from build123d import *

# Parameters (mm, degrees)
SKETCH_W        = 165
SKETCH_H        = 45
PAD_DEPTH       = 22
SKETCH001_W     = 133
SKETCH001_H     = 41
POCKET_DEPTH    = 20
SKETCH002_W     = 26
SKETCH002_H     = 41
POCKET001_DEPTH = 20
SKETCH003_W     = 42
SKETCH003_H     = 47
PAD001_DEPTH    = 2
SKETCH008_W     = 42
SKETCH008_H     = 25
PAD002_DEPTH    = 6
SKETCH005_W     = 30
SKETCH005_H     = 13
POCKET002_DEPTH = 8.001
SKETCH009_R     = 1.5
POCKET003_DEPTH = 8.001
SKETCH007_R     = 2.5
POCKET004_DEPTH = 5


with BuildPart() as part:
    # Sketch → Pad (new body)
    with BuildSketch(Plane.XY):
        with Locations((82.5, 22.5)):
            Rectangle(SKETCH_W, SKETCH_H)
    extrude(amount=PAD_DEPTH)

    # Sketch001 → Pocket (cut)
    with BuildSketch(Plane.XY.offset(22)):
        with Locations((68.54825, 22.488898)):
            Rectangle(SKETCH001_W, SKETCH001_H)
    extrude(amount=-POCKET_DEPTH, mode=Mode.SUBTRACT)

    # Sketch002 → Pocket001 (cut)
    with BuildSketch(Plane.XY.offset(22)):
        with Locations((149.979632, 22.458033)):
            Rectangle(SKETCH002_W, SKETCH002_H)
    extrude(amount=-POCKET001_DEPTH, mode=Mode.SUBTRACT)

    # Sketch003 → Pad001 (new body)
    with BuildSketch(Plane(origin=(0, 45, 0), x_dir=(-1, 0, 0), z_dir=(0, 1, 0))):
        with Locations((-55.599999, 23.509954)):
            Rectangle(SKETCH003_W, SKETCH003_H)
    extrude(amount=PAD001_DEPTH)

    # Sketch008 → Pad002 (new body)
    with BuildSketch(Plane.XZ.offset(-45)):
        with Locations((55.598549, 34.508675)):
            Rectangle(SKETCH008_W, SKETCH008_H)
    extrude(amount=PAD002_DEPTH)

    # Sketch005 → Pocket002 (cut, through all)
    with BuildSketch(Plane.XZ.offset(-39)):
        with Locations((55.035654, 34.372233)):
            Rectangle(SKETCH005_W, SKETCH005_H)
    extrude(amount=-POCKET002_DEPTH, mode=Mode.SUBTRACT)

    # Sketch009 → Pocket003 (cut, through all)
    with BuildSketch(Plane.XZ.offset(-39)):
        with Locations((37.021919, 34.390724)):
            Circle(SKETCH009_R)
        with Locations((72.989189, 34.493778)):
            Circle(SKETCH009_R)
    extrude(amount=-POCKET003_DEPTH, mode=Mode.SUBTRACT)

    # Sketch007 → Pocket004 (cut)
    with BuildSketch(Plane.YZ.offset(165)):
        with Locations((37.952961, 13.56812)):
            Circle(SKETCH007_R)
    extrude(amount=-POCKET004_DEPTH, mode=Mode.SUBTRACT)


solid = part.part
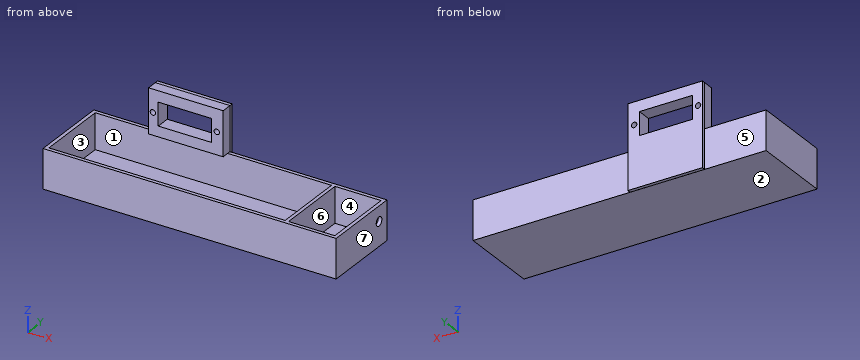
The model under review builds one solid part; all positions refer to its coordinate system, in mm. Face numbers are marked on the shaded views. A direction names the side the tool comes from. Round coordinates to 2 decimals unless told otherwise and drop trailing zeros. Order: outer loops, then holes, each group sorted by start corner. A loop starts at its lowest first (then second) coordinate and runs counter-clockwise, first axis right, second up. Notation, with made-up numbers: (29.5, 75.25) -> (87.5, 75.25) arc R20 ccw to (87.5, 105.25) -> close; hole circle Ø9 at (30.5, -2.75). An arc over 180 degrees is marked (long way). Return JSON: item names as keys, results as strings.
1. For the marked faces 1, 2 and 3, list the 3-axis set-ups (+Z, -Z, +X, -X, +Y, -Y) from which the entire face can be reached by the end or side of a thin tool; tool diameter is ignored.
Answer block:
{"face 1": "none", "face 2": "-Z, +X, -X, +Y, -Y", "face 3": "+Z"}
2. The part is to be moulded in two halves that separate along X. For the marked faces 4, 5, 6 and 7, say which applies: +X half, -X half, draft (parallel to the pull), parting line (faces both ways), or undercut.
Answer block:
{"face 4": "undercut", "face 5": "draft", "face 6": "undercut", "face 7": "+X half"}
3. Insertion check: P1, Ø3, axis at y = 43, z = 36.5, coming from the -X side; P2, Ø22.5, axis at x = 83, y = 12, coming from the +Z side; P3, Ø6.5, axis at y = 43, z = 32.5, coming from the +X side; P4, Ø2, axis at x = 79, z = 24.5, coming from the +Y side. Each pin has a flat end and moves straight along its axis. Give the tip position at first contact, or say it passes through.
Answer block:
{"P1": "stops at x = 34.6", "P2": "stops at z = 22", "P3": "stops at x = 76.6", "P4": "passes through"}
4. For L1, parallel to X at y = 4, z = 9.5; L2, parallel to Y at x = 118.5, z = 6.5; L3, parallel to X at y = 43, z = 40.5, list the stretches that pass through material, from the lowest coordinate up. Write a range as [from, to].
Answer block:
{"L1": "x = [0, 2.05], [135.05, 136.98], [162.98, 165]", "L2": "y = [0, 1.99], [42.99, 45]", "L3": "x = [34.6, 40.04], [70.04, 76.6]"}
5. Take a section at B-B (x = 114.5). Write out the cut boundary in (y, z).
Answer block:
{"outline": "(0, 0) -> (45, 0) -> (45, 22) -> (42.99, 22) -> (42.99, 2) -> (1.99, 2) -> (1.99, 22) -> (0, 22) -> close"}
6. Take a section at D-D (z = 18). Write out the cut boundary in (x, y), then the cut area to 3 significant figures.
Answer block:
{"outline": "(0, 0) -> (165, 0) -> (165, 45) -> (76.6, 45) -> (76.6, 47) -> (34.6, 47) -> (34.6, 45) -> (0, 45) -> close; hole (2.05, 1.99) -> (135.05, 1.99) -> (135.05, 42.99) -> (2.05, 42.99) -> close; hole (136.98, 1.96) -> (162.98, 1.96) -> (162.98, 42.96) -> (136.98, 42.96) -> close", "area": "990 mm²"}
7. Take a section at C-C (y = 37.5). Write out the cut boundary in (x, z).
Answer block:
{"outline": "(0, 0) -> (165, 0) -> (165, 11.11) -> (162.98, 11.11) -> (162.98, 2) -> (136.98, 2) -> (136.98, 22) -> (135.05, 22) -> (135.05, 2) -> (2.05, 2) -> (2.05, 22) -> (0, 22) -> close; (162.98, 16.03) -> (165, 16.03) -> (165, 22) -> (162.98, 22) -> close"}
